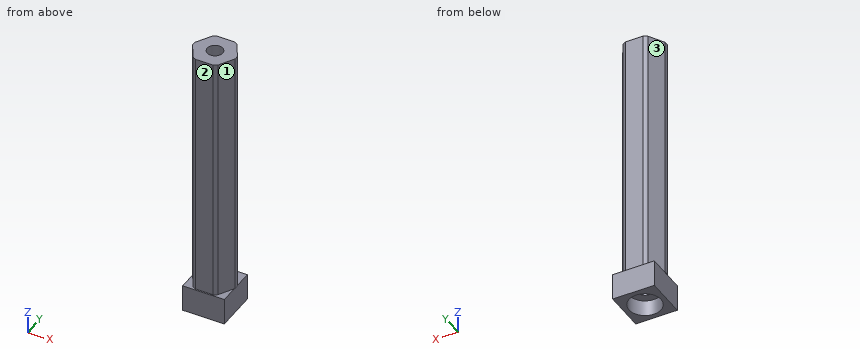
```python
from build123d import *

# Parameters (mm, degrees)
EXTRUDE_1_DEPTH     = 47
SKETCH_2_W          = 7.8
SKETCH_2_H          = 7.8
EXTRUDE_2_DEPTH     = 5
SKETCH_3_R          = 1.45
CUT_EXTRUDE_1_DEPTH = 12.5
SKETCH_4_R          = 3
CUT_EXTRUDE_2_DEPTH = 3
CUT_EXTRUDE_START   = -42.5
SKETCH_3_2_R        = 1.45
CUT_EXTRUDE_3_DEPTH = 9.5


with BuildPart() as part:
    # Эскиз1 → Бобышка-Вытянуть1 (new body)
    with BuildSketch(Plane.XY):
        with BuildLine():
            Line((1.664331698, 3.637306696), (-1.664331698, 3.637306696))
            ThreePointArc((-1.664331698, 3.637306696), (-2, 3.464101615), (-2.317834151, 3.260006878))
            Line((-2.317834151, 3.260006878), (-3.982165849, 0.377299817))
            ThreePointArc((-3.982165849, 0.377299817), (-4, 0), (-3.982165849, -0.377299817))
            Line((-3.982165849, -0.377299817), (-2.317834151, -3.260006878))
            ThreePointArc((-2.317834151, -3.260006878), (-2, -3.464101615), (-1.664331698, -3.637306696))
            Line((-1.664331698, -3.637306696), (1.664331698, -3.637306696))
            ThreePointArc((1.664331698, -3.637306696), (2, -3.464101615), (2.317834151, -3.260006878))
            Line((2.317834151, -3.260006878), (3.982165849, -0.377299817))
            ThreePointArc((3.982165849, -0.377299817), (4, 0), (3.982165849, 0.377299817))
            Line((3.982165849, 0.377299817), (2.317834151, 3.260006878))
            ThreePointArc((2.317834151, 3.260006878), (2, 3.464101615), (1.664331698, 3.637306696))
        make_face()
    extrude(amount=EXTRUDE_1_DEPTH)

    # Эскиз2 → Бобышка-Вытянуть2 (add)
    with BuildSketch(Plane(origin=(0, 0, 0), x_dir=(-1, 0, 0), z_dir=(0, 0, -1))):
        Rectangle(SKETCH_2_W, SKETCH_2_H)
    extrude(amount=EXTRUDE_2_DEPTH)

    # Эскиз3 → Вырез-Вытянуть1 (cut)
    with BuildSketch(Plane(origin=(0, 0, -5), x_dir=(-1, 0, 0), z_dir=(0, 0, -1))):
        Circle(SKETCH_3_R)
    extrude(amount=-CUT_EXTRUDE_1_DEPTH, mode=Mode.SUBTRACT)

    # Эскиз4 → Вырез-Вытянуть2 (cut)
    with BuildSketch(Plane(origin=(0, 0, -5), x_dir=(-1, 0, 0), z_dir=(0, 0, -1))):
        Circle(SKETCH_4_R)
    extrude(amount=-CUT_EXTRUDE_2_DEPTH, mode=Mode.SUBTRACT)

    # Эскиз3<2> → Вырез-Вытянуть3 (cut)
    with BuildSketch(Plane(origin=(0, 0, -5), x_dir=(-1, 0, 0), z_dir=(0, 0, -1)).offset(CUT_EXTRUDE_START)):
        Circle(SKETCH_3_2_R)
    extrude(amount=-CUT_EXTRUDE_3_DEPTH, mode=Mode.SUBTRACT)


solid = part.part
```
Verification items for the finished model (mm, model axes). Face numbers are marked on the shaded views. A direction names the side the tool comes from. Round coordinates to 2 decimals unless told otherwise and drop trailing zeros. Write each loop counter-clockwise with the first axis right and the second up, starting at its lowest first coordinate (ties: lowest second). Pieces come first, ordered by that corner, then holes. Notation, with made-up numbers: (58.25, -10) -> (88.25, -10) arc R38 ccw to (88.25, 28) -> close; hole circle Ø1 at (30.25, 68). An arc over 180 degrees is marked (long way). Write each question's results on one line, items separated by ' | '. Start each with the question number.
1. Cross-section at A-A (z = 38). Enter the section's corners in (x, y).
2. Cross-section at B-B (x = 0). Enter the section's corners in (y, z).
3. Depth check by flat-ended pin: P1, Ø2.5, axis at y = -2, z = -2, coming from the +X side; P2, Ø4, axis at y = -1, z = -2, coming from the -X side; P3, Ø2.5, axis at x = -0.5, y = 0, coming from the -Z side. Enter the tip coordinate at first touch or a pass-through.
4. Set-up check for the marked faces 1, 2 and 3: record each of +Z, -Z, +X, -X, +Y, -Y from which the full face is reachable in a straight line by a thin tool's end or side.
5. Cross-section at D-D (y = 2.5). Enter the section's corners in (x, z).
6. Material ranges on probe 1 along Y at (x, z) = (0, 40.75); probe 2 along Y at (x, z) = (-0.5, 24); probe 3 along X at (y, z) = (0.25, 23.5), recorded low to high. Write a range as from..to.
7. Cross-section at C-C (z = 19). Enter the section's corners in (x, y).
Solutions:
1) outline: (-3.98, -0.38) -> (-2.32, -3.26) arc R4 ccw to (-1.66, -3.64) -> (1.66, -3.64) arc R4 ccw to (2.32, -3.26) -> (3.98, -0.38) arc R4 ccw to (3.98, 0.38) -> (2.32, 3.26) arc R4 ccw to (1.66, 3.64) -> (-1.66, 3.64) arc R4 ccw to (-2.32, 3.26) -> (-3.98, 0.38) arc R4 ccw to start; hole circle Ø2.9 at (0, 0)
2) outline: (-3.9, -5) -> (-3, -5) -> (-3, -2) -> (-1.45, -2) -> (-1.45, 7.5) -> (1.45, 7.5) -> (1.45, -2) -> (3, -2) -> (3, -5) -> (3.9, -5) -> (3.9, 0) -> (3.64, 0) -> (3.64, 47) -> (1.45, 47) -> (1.45, 37.5) -> (-1.45, 37.5) -> (-1.45, 47) -> (-3.64, 47) -> (-3.64, 0) -> (-3.9, 0) -> close
3) P1: stops at x = 3.9 | P2: stops at x = -3.9 | P3: stops at z = -2
4) face 1: +Z, +X, -Y | face 2: +Z, +X, -X, -Y | face 3: +Z, -X, +Y
5) outline: (-3.9, -5) -> (-1.66, -5) -> (-1.66, -2) -> (1.66, -2) -> (1.66, -5) -> (3.9, -5) -> (3.9, 0) -> (2.76, 0) -> (2.76, 47) -> (-2.76, 47) -> (-2.76, 0) -> (-3.9, 0) -> close
6) probe 1: y = -3.64..-1.45, 1.45..3.64 | probe 2: y = -3.64..3.64 | probe 3: x = -3.99..3.99
7) outline: (-3.98, -0.38) -> (-2.32, -3.26) arc R4 ccw to (-1.66, -3.64) -> (1.66, -3.64) arc R4 ccw to (2.32, -3.26) -> (3.98, -0.38) arc R4 ccw to (3.98, 0.38) -> (2.32, 3.26) arc R4 ccw to (1.66, 3.64) -> (-1.66, 3.64) arc R4 ccw to (-2.32, 3.26) -> (-3.98, 0.38) arc R4 ccw to start
